Geometry check sheet. Reference: drawing and pictorial views, mm from the part's lowest x, y, z. Round coordinates to 2 decimals unless told otherwise and drop trailing zeros. Loops run counter-clockwise (first coordinate to the right, second up) from the corner with the lowest first, then second, coordinate; pieces in that order, holes last. Notation, with made-up numbers: (-11.75, 21.5) - (31.25, 21.5) arc R13 ccw to (31.25, 27.5) - close; hole circle Ø8 at (21, -19). An arc over 180 degrees is marked (long way). Return JSON: item names as keys, results as strings.
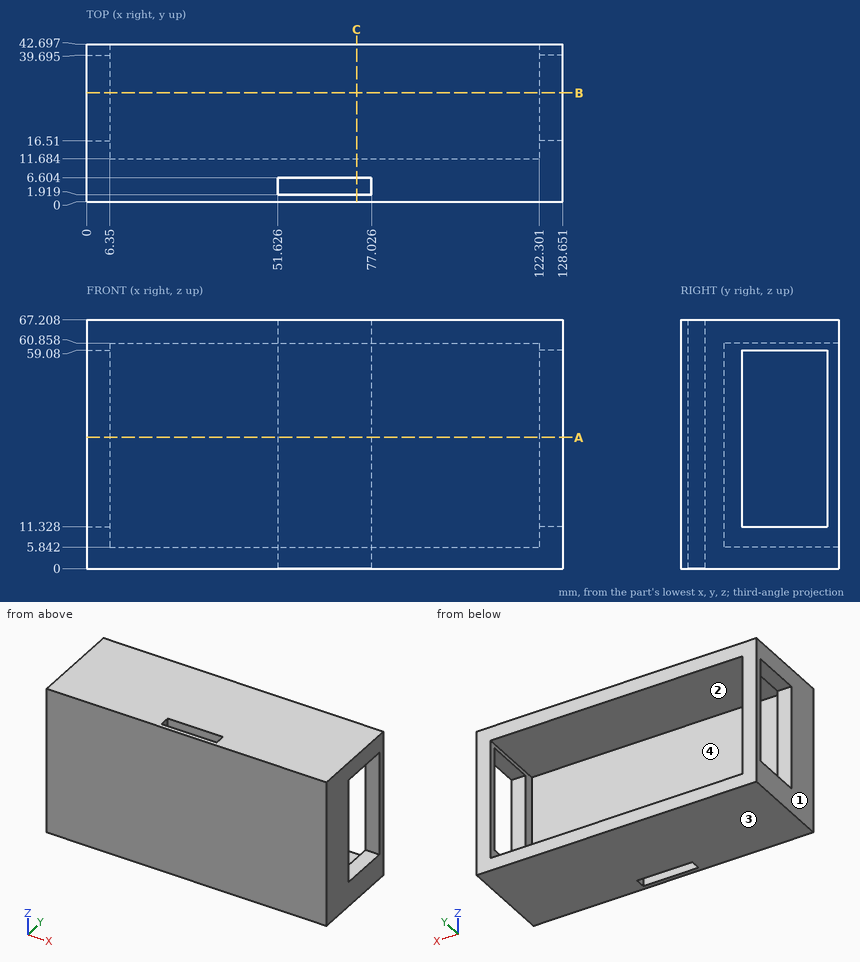
Q1. Sectioned sample at A-A (z = 35.5). State how many separate pieces and enclosed holes the cut face has, plus the area to 3 significant figures.
Answer key:
{"separate pieces": "3", "enclosed holes": "1", "area": "1,480 mm²"}
Q2. Draft check along Z on the marked faces 1, 2, 3 and 4. Enter one of: released by +Z, released by -Z, zero draft, split by the parting line, or undercut.
Answer key:
{"face 1": "zero draft", "face 2": "undercut", "face 3": "released by -Z", "face 4": "undercut"}
Q3. Depth check by flat-ended pin: P1, Ø7.5, axis at x = 63, z = 22.5, coming from the -Y side; P2, Ø8, axis at x = 27.5, z = 33, coming from the +Y side. Enter the tip coordinate at first touch or a pass-through.
Answer key:
{"P1": "stops at y = 0", "P2": "stops at y = 11.68"}
Q4. Scan lines: probe 1 along Z at (x, y) = (66, 25.5); probe 2 along X at (y, z) = (15.5, 14); probe 3 along Y at (x, z) = (61.5, 39) (1 decimal). Record each from-to range of solid material in increasing order. Write a range as [from, to].
Answer key:
{"probe 1": "z = [0, 5.84], [60.86, 67.21]", "probe 2": "x = [0, 6.35], [122.3, 128.65]", "probe 3": "y = [0, 1.9], [6.6, 11.7]"}
Q5. Sectioned sample at C-C (x = 73). Enter the section's corners in (y, z) (1 decimal).
Answer key:
{"outline": "(0, 0) - (1.9, 0) - (1.9, 67.2) - (0, 67.2) - close; (6.6, 0) - (42.7, 0) - (42.7, 5.8) - (11.7, 5.8) - (11.7, 60.9) - (42.7, 60.9) - (42.7, 67.2) - (6.6, 67.2) - close"}
Q6. Sectioned sample at B-B (y = 29.5). Enter the section's corners in (x, z), plus the area to 3 significant figures.
Answer key:
{"outline": "(0, 0) - (128.65, 0) - (128.65, 11.33) - (122.3, 11.33) - (122.3, 5.84) - (6.35, 5.84) - (6.35, 11.33) - (0, 11.33) - close; (0, 59.08) - (6.35, 59.08) - (6.35, 60.86) - (122.3, 60.86) - (122.3, 59.08) - (128.65, 59.08) - (128.65, 67.21) - (0, 67.21) - close", "area": "1,660 mm²"}
